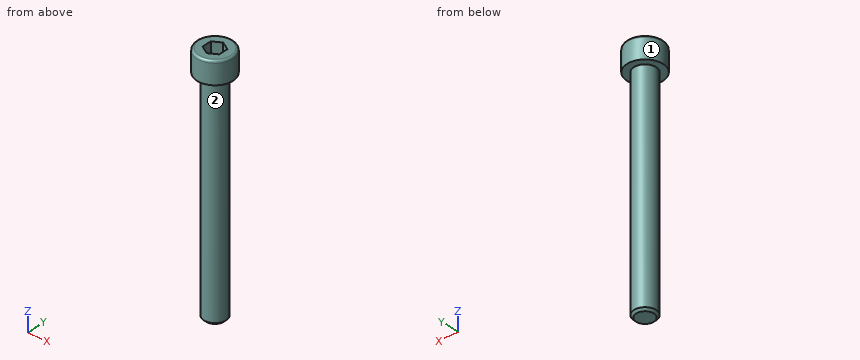
from build123d import *

# Parameters (mm, degrees)
ODEBR_N_PROTA_EN_1_DEPTH = 6


with BuildPart() as part:
    # Skica1 → Základ-Rotační (revolve)
    with BuildSketch(Plane(origin=(0, 0, 0), x_dir=(1, 0, 0), z_dir=(0, 1, 0))):
        with BuildLine():
            Line((0, 80), (0, -8))
            Line((0, -8), (5.7, -8))
            ThreePointArc((5.7, -8), (6.265685425, -7.765685425), (6.5, -7.2))
            Line((6.5, -7.2), (6.5, 0))
            Line((6.5, 0), (4, 0))
            Line((4, 0), (4, 79.2))
            Line((4, 79.2), (3.2, 80))
            Line((3.2, 80), (0, 80))
        make_face()
    revolve(axis=Axis((0, 0, -20.555484665), (0, 0, -1)))

    # Skica2 → Odebrání-Protažení1 (cut)
    with BuildSketch(Plane.XY.offset(8)):
        Polygon((3, -1.732050808), (3, 1.732050808), (0, 3.464101615), (-3, 1.732050808), (-3, -1.732050808), (0, -3.464101615), align=None)
    extrude(amount=-ODEBR_N_PROTA_EN_1_DEPTH, mode=Mode.SUBTRACT)


solid = part.part
Design review of the part built by this model. Coordinates are the model's own, in mm. Face numbers are marked on the shaded views. A direction names the side the tool comes from. Give positions to 0.01 mm unless a question says otherwise; leave off trailing zeros. Write each loop counter-clockwise with the first axis right and the second up, starting at its lowest first coordinate (ties: lowest second). Pieces come first, ordered by that corner, then holes. Notation, with made-up numbers: M -6.75,-23 L 10.25,-23 A18 cw 10.25,-14 Z; hole C 44.5,19.5 d11. An arc over 180 degrees is marked long. Answer as a JSON object with one key per item and string values. Group by question number.
1) We need section B-B (z = -18). Give the boundary of the cut face in (x, y).
2) Tool access review of the marked faces 1 and 2: name each direction out of +Z, -Z, +X, -X, +Y, -Y from which nothing blocks a thin tool from reaching the whole face with its end or side.
3) Clearance check with flat-ended pins moving along their axes: pin 1 Ø1 at (x, z) = (-0.5, -22.5) entering from -Y; pin 2 Ø3 at (x, y) = (-0.5, -0.5) entering from +Z; pin 3 Ø5 at (x, z) = (0, -48.5) entering from +Y. State where each tip first meets the part, or that it passes through.
4) For line 1 along Z through (x, y) = (-1.25, 1.5); line 2 along X through (y, z) = (-2, -63); line 3 along Y through (x, z) = (0, -21.5), list the stretches that pass through material, from the lowest coordinate up.
5) We need section A-A (y = 0). Give the boundary of the cut face in (x, z), and give its area (3 significant figures).
Answer key:
{
 "1": {"outline": "C 0,0 d8"},
 "2": {"face 1": "+Z, -Z", "face 2": "-Z"},
 "3": {"pin 1": "stops at y = -4", "pin 2": "stops at z = 2", "pin 3": "stops at y = 4"},
 "4": {"line 1": "z = -80 to 2", "line 2": "x = -3.46 to 3.46", "line 3": "y = -4 to 4"},
 "5": {"outline": "M -6.5,0 L -4,0 L -4,-79.2 L -3.2,-80 L 3.2,-80 L 4,-79.2 L 4,0 L 6.5,0 L 6.5,7.2 A0.8 ccw 5.7,8 L 3,8 L 3,2 L -3,2 L -3,8 L -5.7,8 A0.8 ccw -6.5,7.2 Z", "area": "707 mm²"}
}
